The listing builds one solid part. Answer for the finished solid, in the listing's coordinates (mm). A direction names the side the tool comes from. Round coordinates to 2 decimals unless told otherwise and drop trailing zeros. Loops run counter-clockwise (first coordinate to the right, second up) from the corner with the lowest first, then second, coordinate; pieces in that order, holes last. Notation, with made-up numbers: (-3.75, 34.5) -> (20.25, 34.5) arc R9 ccw to (20.25, 47.5) -> close; hole circle Ø2 at (47.5, 4). An arc over 180 degrees is marked (long way). Write each question's results on one line, items separated by ' | '. Start each with the question number.
(1) Determine the mould class of faces 1 (the face through (126.885, -57.749, -13.063)), 2 (the face through (111.753, 3.621, -34.279)), 3 (the face through (27, 18, -17.5)), 4 (the face through (125, -66, -13)) for opening direction Y: released by +Y, released by -Y, zero draft, split by the parting line, or undercut.
(2) The part is cut by section B-B (y = -18.5). Determine the outline of the cut face in (x, z), plus the area to 3 significant figures.
(3) Flat-ended cylindrical pins translate along their axes: pin 1 (3 mm diameter, centred on y = 11.5, z = -21, fed in from +X); pin 2 (2 mm diameter, centred on x = 93, y = 17, fed in from -Z); pin 3 (2.5 mm diameter, centred on x = 50.5, y = 5.5, fed in from -Z); pin 4 (4 mm diameter, centred on x = 7.5, y = -58.5, fed in from -Z). Find the tip coordinate at first contact, or state that the pin passes through.
(4) For faces 5 (the face through (91.753, 3.621, -34.279)), 6 (the face through (105, 18, -17.5)), 7 (the face through (84.5, 13, -21)), 8 (the face through (38, 17, -32.5)), determine the directions among +Z, -Z, +X, -X, +Y, -Y from which every point of the face is accessible in a straight line to the end or side of a thin tool.
(5) Straight lines are drawn through the part: probe 1 along Y at (x, z) = (7.5, -12.5); probe 2 along Y at (x, z) = (124, -14); probe 3 along X at (y, z) = (-39, -10). For each, find the intervals that lie inside material, in ascending order.
(6) The part is cut by section A-A (y = -53.5). Determine the outline of the cut face in (x, z), plus the area to 3 significant figures.
(7) The part is cut by section C-C (y = 3.5). Determine the outline of the cut face in (x, z), plus the area to 3 significant figures.
(8) The part is cut by section D-D (x = 24.5). Determine the outline of the cut face in (y, z).
```python
from build123d import *

# Parameters (mm, degrees)
BOSS_EXTRUDE2_START  = -1
SKETCH1_W            = 66
SKETCH1_H            = 19
BOSS_EXTRUDE2_DEPTH  = 9
SKETCH3_R            = 2.75
BOSS_EXTRUDE3_DEPTH  = 13.75
SKETCH4_W            = 4.5
SKETCH4_H            = 6.5
BOSS_EXTRUDE4_DEPTH  = 15
BOSS_EXTRUDE5_DEPTH  = 8.5
SKETCH8_W            = 9
SKETCH8_H            = 6.5
BOSS_EXTRUDE6_DEPTH  = 6
SKETCH9_W            = 15.5
SKETCH9_H            = 6.5
BOSS_EXTRUDE7_DEPTH  = 21
BOSS_EXTRUDE8_DEPTH  = 8.5
CUT_EXTRUDE2_START   = -8.5
SKETCH12_R           = 3.5
CUT_EXTRUDE2_DEPTH   = 8.5
FILLET1_R            = 10
SKETCH14_W           = 15
SKETCH14_H           = 9
BOSS_EXTRUDE10_DEPTH = 65
CUT_EXTRUDE3_REACH   = 98.312
SKETCH15_R           = 2.5
FILLET1_OF_MIRROR3_R = 10


with BuildPart() as part:
    # Sketch1 → Boss-Extrude2 (new body)
    with BuildSketch(Plane(origin=(0, 0, 0), x_dir=(1, 0, 0), z_dir=(0, 1, 0)).offset(BOSS_EXTRUDE2_START)):
        with Locations((33, 18)):
            Rectangle(SKETCH1_W, SKETCH1_H)
    boss_extrude2 = extrude(amount=BOSS_EXTRUDE2_DEPTH)

    # Sketch3 → Boss-Extrude3 (add)
    with BuildSketch(Plane(origin=(0, 0, -27.5), x_dir=(-1, 0, 0), z_dir=(0, 0, -1))):
        with Locations((-37.5, 3.5)):
            Circle(SKETCH3_R)
        with Locations((-17.5, 3.5)):
            Circle(SKETCH3_R)
    boss_extrude3 = extrude(amount=BOSS_EXTRUDE3_DEPTH)

    # Sketch4 → Boss-Extrude4 (add)
    with BuildSketch(Plane(origin=(0, 8, 0), x_dir=(1, 0, 0), z_dir=(0, 1, 0))):
        with Locations((25.25, 20.75)):
            Rectangle(SKETCH4_W, SKETCH4_H)
        with Locations((29.75, 20.75)):
            Rectangle(SKETCH4_W, SKETCH4_H)
    boss_extrude4 = extrude(amount=BOSS_EXTRUDE4_DEPTH)

    # Sketch5 → Boss-Extrude5 (add)
    with BuildSketch(Plane(origin=(0, 0, -24), x_dir=(-1, 0, 0), z_dir=(0, 0, -1))):
        with BuildLine():
            ThreePointArc((-25.636419782, 13.037388184), (-24.436298745, 14.307742745), (-24, 16))
            ThreePointArc((-24, 16), (-29.974873734, 18.474873734), (-27.5, 12.5))
            ThreePointArc((-27.5, 12.5), (-26.685966178, 12.595980474), (-25.916578842, 12.878657751))
            ThreePointArc((-25.916578842, 12.878657751), (-25.85405917, 13.094916041), (-25.636419782, 13.037388184))
        make_face()
    extrude(amount=BOSS_EXTRUDE5_DEPTH)

    # Sketch8 → Boss-Extrude6 (add)
    with BuildSketch(Plane(origin=(0, 23, 0), x_dir=(1, 0, 0), z_dir=(0, 1, 0))):
        with Locations((27.5, 20.75)):
            Rectangle(SKETCH8_W, SKETCH8_H)
    boss_extrude6 = extrude(amount=BOSS_EXTRUDE6_DEPTH)

    # Sketch9 → Boss-Extrude7 (add)
    with BuildSketch(Plane(origin=(0, 8, 0), x_dir=(1, 0, 0), z_dir=(0, 1, 0))):
        with Locations((39.75, 20.75)):
            Rectangle(SKETCH9_W, SKETCH9_H)
        with Locations((15.25, 20.75)):
            Rectangle(SKETCH9_W, SKETCH9_H)
    boss_extrude7 = extrude(amount=BOSS_EXTRUDE7_DEPTH)

    # Sketch10 → Boss-Extrude8 (add)
    with BuildSketch(Plane(origin=(0, 0, -24), x_dir=(-1, 0, 0), z_dir=(0, 0, -1))):
        with BuildLine():
            Line((-21, 17), (-17.5, 17))
            Line((-17.5, 17), (-14, 17))
            ThreePointArc((-14, 17), (-17.5, 20.5), (-21, 17))
        make_face()
        with BuildLine():
            Line((-17.5, 13.5), (-17.5, 17))
            Line((-17.5, 17), (-21, 17))
            ThreePointArc((-21, 17), (-19.974873734, 14.525126266), (-17.5, 13.5))
        make_face()
        with BuildLine():
            Line((-14, 17), (-17.5, 17))
            Line((-17.5, 17), (-17.5, 13.5))
            ThreePointArc((-17.5, 13.5), (-15.025126266, 14.525126266), (-14, 17))
        make_face()
        with BuildLine():
            Line((-37.5, 17), (-34, 17))
            ThreePointArc((-34, 17), (-37.5, 20.5), (-41, 17))
            Line((-41, 17), (-37.5, 17))
        make_face()
        with BuildLine():
            ThreePointArc((-37.5, 13.5), (-35.025126266, 14.525126266), (-34, 17))
            Line((-34, 17), (-37.5, 17))
            Line((-37.5, 17), (-37.5, 13.5))
        make_face()
        with BuildLine():
            Line((-37.5, 13.5), (-37.5, 17))
            Line((-37.5, 17), (-41, 17))
            ThreePointArc((-41, 17), (-39.974873734, 14.525126266), (-37.5, 13.5))
        make_face()
    boss_extrude8 = extrude(amount=BOSS_EXTRUDE8_DEPTH)

    # Sketch12 → Cut-Extrude2 (cut)
    with BuildSketch(Plane(origin=(0, 0, -32.5), x_dir=(-1, 0, 0), z_dir=(0, 0, -1)).offset(CUT_EXTRUDE2_START)):
        with Locations((-27.5, 16)):
            Circle(SKETCH12_R)
    extrude(amount=CUT_EXTRUDE2_DEPTH, mode=Mode.SUBTRACT)

    # Fillet1
    fillet1_edges = [part.edges().sort_by_distance(p)[0] for p in [
        (7.5, 29, -20.75),
        (47.5, 29, -20.75),
    ]]
    fillet(fillet1_edges, radius=FILLET1_R)

    # Sketch14 → Boss-Extrude10 (add)
    with BuildSketch(Plane.XZ.offset(1)):
        with Locations((7.5, -13)):
            Rectangle(SKETCH14_W, SKETCH14_H)
    boss_extrude10 = extrude(amount=BOSS_EXTRUDE10_DEPTH)

    # Sketch15 → Cut-Extrude3 (cut, up to next)
    with BuildSketch(Plane(origin=(0, 0, -17.5), x_dir=(-1, 0, 0), z_dir=(0, 0, -1)), mode=Mode.PRIVATE) as cut_extrude3_sk1:
        with Locations((-7.5, -18.5)):
            Circle(SKETCH15_R)
    cut_extrude3_tool1 = extrude(cut_extrude3_sk1.sketch, amount=-CUT_EXTRUDE3_REACH, mode=Mode.PRIVATE) & part.part
    # Sketch15 → Cut-Extrude3 (cut, up to next)
    with BuildSketch(Plane(origin=(0, 0, -17.5), x_dir=(-1, 0, 0), z_dir=(0, 0, -1)), mode=Mode.PRIVATE) as cut_extrude3_sk2:
        with Locations((-7.5, -58.5)):
            Circle(SKETCH15_R)
    cut_extrude3_tool2 = extrude(cut_extrude3_sk2.sketch, amount=-CUT_EXTRUDE3_REACH, mode=Mode.PRIVATE) & part.part
    cut_extrude3_1 = cut_extrude3_tool1.solids().sort_by_distance((7.5, -18.5, -17.5))[0]
    add(cut_extrude3_1, mode=Mode.SUBTRACT)
    cut_extrude3_2 = cut_extrude3_tool2.solids().sort_by_distance((7.5, -58.5, -17.5))[0]
    add(cut_extrude3_2, mode=Mode.SUBTRACT)
    cut_extrude3 = cut_extrude3_1 + cut_extrude3_2  # Cut-Extrude3 as one shape, for the pattern or mirror that repeats it

    # Mirror3: Boss-Extrude2, Boss-Extrude3, Boss-Extrude4, Boss-Extrude6, Boss-Extrude7, Boss-Extrude8, Boss-Extrude10, Cut-Extrude3 across plane
    add(boss_extrude2.mirror(Plane(origin=(66, -1, -8.5), x_dir=(0, 0, 1), z_dir=(1, 0, 0))))
    add(boss_extrude3.mirror(Plane(origin=(66, -1, -8.5), x_dir=(0, 0, 1), z_dir=(1, 0, 0))))
    add(boss_extrude4.mirror(Plane(origin=(66, -1, -8.5), x_dir=(0, 0, 1), z_dir=(1, 0, 0))))
    add(boss_extrude6.mirror(Plane(origin=(66, -1, -8.5), x_dir=(0, 0, 1), z_dir=(1, 0, 0))))
    add(boss_extrude7.mirror(Plane(origin=(66, -1, -8.5), x_dir=(0, 0, 1), z_dir=(1, 0, 0))))
    add(boss_extrude8.mirror(Plane(origin=(66, -1, -8.5), x_dir=(0, 0, 1), z_dir=(1, 0, 0))))
    add(boss_extrude10.mirror(Plane(origin=(66, -1, -8.5), x_dir=(0, 0, 1), z_dir=(1, 0, 0))))
    add(cut_extrude3.mirror(Plane(origin=(66, -1, -8.5), x_dir=(0, 0, 1), z_dir=(1, 0, 0))), mode=Mode.SUBTRACT)

    # Fillet1 of Mirror3
    fillet1_of_mirror3_edges = [part.edges().sort_by_distance(p)[0] for p in [
        (124.5, 29, -20.75),
        (84.5, 29, -20.75),
    ]]
    fillet(fillet1_of_mirror3_edges, radius=FILLET1_OF_MIRROR3_R)


solid = part.part
```
Checked values:
1) face 1: undercut | face 2: undercut | face 3: zero draft | face 4: released by -Y
2) outline: (0, -17.5) -> (5, -17.5) -> (5, -8.5) -> (0, -8.5) -> close; (10, -17.5) -> (15, -17.5) -> (15, -8.5) -> (10, -8.5) -> close; (117, -17.5) -> (122, -17.5) -> (122, -8.5) -> (117, -8.5) -> close; (127, -17.5) -> (132, -17.5) -> (132, -8.5) -> (127, -8.5) -> close | area: 180 mm2
3) pin 1: stops at x = 124.5 | pin 2: stops at z = -32.5 | pin 3: stops at z = -27.5 | pin 4: passes through
4) face 5: -Z | face 6: +Z, +X, -X, +Y | face 7: +Z, -Z, +Y | face 8: -Z, +X, -X, +Y
5) probe 1: y = -66 to -61, -56 to -21, -16 to 8 | probe 2: y = -66 to -60.95, -56.05 to -20.95, -16.05 to 8 | probe 3: x = 0 to 15, 117 to 132
6) outline: (0, -17.5) -> (15, -17.5) -> (15, -8.5) -> (0, -8.5) -> close; (117, -17.5) -> (132, -17.5) -> (132, -8.5) -> (117, -8.5) -> close | area: 270 mm2
7) outline: (0, -27.5) -> (14.75, -27.5) -> (14.75, -41.25) -> (20.25, -41.25) -> (20.25, -27.5) -> (34.75, -27.5) -> (34.75, -41.25) -> (40.25, -41.25) -> (40.25, -27.5) -> (91.75, -27.5) -> (91.75, -41.25) -> (97.25, -41.25) -> (97.25, -27.5) -> (111.75, -27.5) -> (111.75, -41.25) -> (117.25, -41.25) -> (117.25, -27.5) -> (132, -27.5) -> (132, -8.5) -> (0, -8.5) -> close | area: 2,810 mm2
8) outline: (-1, -27.5) -> (8, -27.5) -> (8, -24) -> (29, -24) -> (29, -17.5) -> (8, -17.5) -> (8, -8.5) -> (-1, -8.5) -> close
